from build123d import *

# Parameters (mm, degrees)
SKETCH_1_W          = 8.8
SKETCH_1_H          = 4.6
EXTRUDE_1_DEPTH     = 4.7
SKETCH_1_3_W        = 4.2
SKETCH_1_3_H        = 2.2
SKETCH_1_3_W_2      = 2
SKETCH_1_3_H_2      = 2
CUT_EXTRUDE_1_DEPTH = 0.2
SKETCH_1_4_W        = 2
SKETCH_1_4_H        = 2
EXTRUDE_2_DEPTH     = 2
SKETCH_2_R          = 0.2
SKETCH_2_W          = 0.4
SKETCH_2_H          = 1.2
EXTRUDE_3_DEPTH     = 3.3


with BuildPart() as part:
    # Sketch 1 → Extrude 1 (new body)
    with BuildSketch(Plane.XY):
        with Locations((4.4, -2.3)):
            Rectangle(SKETCH_1_W, SKETCH_1_H)
    extrude(amount=EXTRUDE_1_DEPTH)

    # Sketch 1_3 → Cut-Extrude 1 (cut)
    with BuildSketch(Plane.XY):
        with Locations((4.4, -2.3)):
            Rectangle(SKETCH_1_3_W, SKETCH_1_3_H)
        with Locations((3.4, -2.3)):
            Rectangle(SKETCH_1_3_W_2, SKETCH_1_3_H_2, mode=Mode.SUBTRACT)
    extrude(amount=CUT_EXTRUDE_1_DEPTH, mode=Mode.SUBTRACT)

    # Sketch 1_4 → Extrude 2 (add)
    with BuildSketch(Plane.XY):
        with Locations((3.4, -2.3)):
            Rectangle(SKETCH_1_4_W, SKETCH_1_4_H)
    extrude(amount=-EXTRUDE_2_DEPTH)

    # Sketch 2 → Extrude 3 (add)
    with BuildSketch(Plane.XY.offset(4.7)):
        with Locations(Location((2.4, -2.3, 0), (0, 0, 180))):
            Circle(SKETCH_2_R)
        with Locations(Location((4.4, -2.3, 0), (0, 0, 180))):
            Circle(SKETCH_2_R)
        with Locations(Location((6.4, -2.3, 0), (0, 0, 180))):
            Circle(SKETCH_2_R)
        with Locations((8.6, -2.3)):
            Rectangle(SKETCH_2_W, SKETCH_2_H)
        with Locations((0.2, -2.3)):
            Rectangle(SKETCH_2_W, SKETCH_2_H)
    extrude(amount=EXTRUDE_3_DEPTH)


solid = part.part
Build history of the part. All positions in model axes, mm. A direction names the side the tool comes from. Give positions to 0.01 mm unless a question says otherwise; leave off trailing zeros. Order: outer loops, then holes, each group sorted by start corner. A loop starts at its lowest first (then second) coordinate and runs counter-clockwise, first axis right, second up. Notation, with made-up numbers: M -40,89.5 L -36,89.5 A32 cw -36,117.5 Z; hole C 46,29.25 d9. An arc over 180 degrees is marked long. Put each result on its own line as item: value.
Item 1: Slice it at D-D, the plane z = -0.25. Write the cut outline in (x, y).
From the geometry:
outline: M 2.4,-3.3 L 4.4,-3.3 L 4.4,-1.3 L 2.4,-1.3 Z
Item 2: Probe line 1 (X direction, y = -1.75, z = 7.5); line 2 (Z direction, x = 2.5, y = -2.8); line 3 (Z direction, x = 8.5, y = -0.9). List the from-to ranges inside material, lowest first. Write a range as [from, to].
From the geometry:
line 1: x = [0, 0.4], [8.4, 8.8]
line 2: z = [-2, 4.7]
line 3: z = [0, 4.7]
Item 3: Slice it at A-A, the plane z = 5.5. Write the cut outline in (x, y), plus the area to 3 significant figures.
From the geometry:
outline: M 0,-2.9 L 0.4,-2.9 L 0.4,-1.7 L 0,-1.7 Z; C 2.4,-2.3 d0.4; C 4.4,-2.3 d0.4; C 6.4,-2.3 d0.4; M 8.4,-2.9 L 8.8,-2.9 L 8.8,-1.7 L 8.4,-1.7 Z
area: 1.34 mm2
Item 4: Two-plate mould, pull along X, no slides. Class faces 3 (the flat face through (8.8, -2, 3)), 4 (the flat face through (4, -3, 4.7)), 5 (the flat face through (0, -2, 3)), 6 (the flat face through (4, 0, 2)): +X half, -X half, draft (parallel to the pull), parting line (faces both ways), or undercut.
From the geometry:
face 3: +X half
face 4: undercut
face 5: -X half
face 6: draft
Item 5: 3-axis set-ups, long thin cutter, end or side, ignore diameter. For faces 1 (the flat face through (8.4, -2, 6)), 2 (the flat face through (3, -2, -2)): which of +Z, -Z, +X, -X, +Y, -Y reach the whole face in a straight line?
From the geometry:
face 1: +Z, +Y, -Y
face 2: -Z, +X, -X, +Y, -Y
Item 6: Flat gauge pins, fed straight in: pin 1 Ø1.6 at (x, z) = (3.5, -1) entering from -Y; pin 2 Ø1.1 at (x, y) = (5.5, -2.5) entering from -Z; pin 3 Ø0.6 at (y, z) = (-2.5, -1.5) entering from -X. Where does each tip first touch, or does it go through?
From the geometry:
pin 1: stops at y = -3.3
pin 2: stops at z = 0.2
pin 3: stops at x = 2.4
Item 7: Slice it at B-B, the plane y = -3.05. Write the cut outline in (x, z), plus the area to 3 significant figures.
From the geometry:
outline: M 0,0 L 2.3,0 L 2.3,0.2 L 2.4,0.2 L 2.4,-2 L 4.4,-2 L 4.4,0.2 L 6.5,0.2 L 6.5,0 L 8.8,0 L 8.8,4.7 L 0,4.7 Z
area: 44.9 mm2
Item 8: Slice it at C-C, the plane x = 4.75. Write the cut outline in (y, z).
From the geometry:
outline: M -4.6,0 L -3.4,0 L -3.4,0.2 L -1.2,0.2 L -1.2,0 L 0,0 L 0,4.7 L -4.6,4.7 Z
